from build123d import *

# Parameters (mm, degrees)
SKETCH1_R           = 125
SKETCH1_W           = 175
SKETCH1_H           = 95
BOSS_EXTRUDE1_DEPTH = 3
SKETCH2_R           = 3.25
SKETCH2_R_2         = 3
CUT_EXTRUDE1_DEPTH  = 4


with BuildPart() as part:
    # Sketch1 → Boss-Extrude1 (new body)
    with BuildSketch(Plane.XY):
        Circle(SKETCH1_R)
        Rectangle(SKETCH1_W, SKETCH1_H, mode=Mode.SUBTRACT)
    extrude(amount=BOSS_EXTRUDE1_DEPTH)

    # Sketch2 → Cut-Extrude1 (cut, through all)
    with BuildSketch(Plane.XY.offset(3)):
        with Locations((-52, -64.5)):
            Circle(SKETCH2_R)
        with Locations((-55, -93.5)):
            Circle(SKETCH2_R_2)
        with Locations((52, 64.5)):
            Circle(SKETCH2_R)
        with Locations((55, 93.5)):
            Circle(SKETCH2_R_2)
        with Locations((52, -64.5)):
            Circle(SKETCH2_R)
        with Locations((-52, 64.5)):
            Circle(SKETCH2_R)
        with Locations((49, -93.5)):
            Circle(SKETCH2_R)
        with Locations((-49, 93.5)):
            Circle(SKETCH2_R)
    extrude(amount=-CUT_EXTRUDE1_DEPTH, mode=Mode.SUBTRACT)


solid = part.part
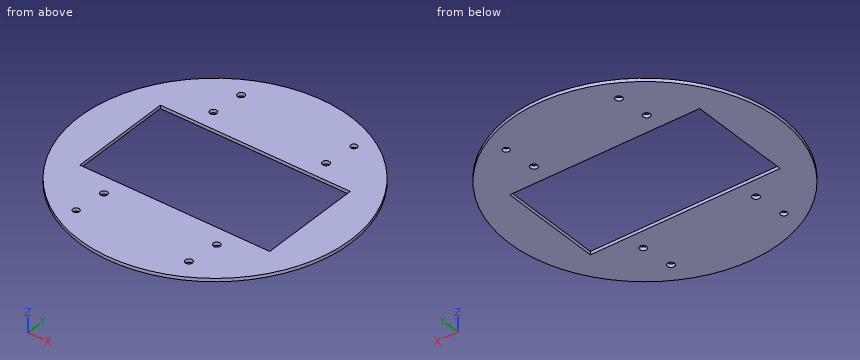
Part model, mm, in its own coordinate system. Give positions to 0.01 mm unless a question says otherwise; leave off trailing zeros. Loops run counter-clockwise (first coordinate to the right, second up) from the corner with the lowest first, then second, coordinate; pieces in that order, holes last.
(1) Band-saw the part on D-D (y = 93.5). Write the cut outline in (x, z), and give its area (3 significant figures).
Return value:
outline: (-82.96, 0) - (-52.25, 0) - (-52.25, 3) - (-82.96, 3) - close; (-45.75, 0) - (52, 0) - (52, 3) - (-45.75, 3) - close; (58, 0) - (82.96, 0) - (82.96, 3) - (58, 3) - close
area: 460 mm2
(2) Drill centre lines: line 1 along Y through (x, z) = (-1.5, 0.3); line 2 along Y through (x, z) = (-55, 2.1); line 3 along Y through (x, z) = (55, 1.95). Where is each one in solid material? Low to high.
Return value:
line 1: y = -124.99 to -47.5, 47.5 to 124.99
line 2: y = -112.25 to -96.5, -90.5 to -65.75, -63.25 to -47.5, 47.5 to 63.25, 65.75 to 112.25
line 3: y = -112.25 to -65.75, -63.25 to -47.5, 47.5 to 63.25, 65.75 to 90.5, 96.5 to 112.25
(3) Band-saw the part on B-B (z = 2). Count the separate pieces of the cut face and the enclosed holes in it, and give its area (3 significant figures).
Return value:
separate pieces: 1
enclosed holes: 9
area: 32,200 mm2
(4) Band-saw the part on A-A (y = 44). Write the cut outline in (x, z), and give its area (3 significant figures).
Return value:
outline: (-117, 0) - (-87.5, 0) - (-87.5, 3) - (-117, 3) - close; (87.5, 0) - (117, 0) - (117, 3) - (87.5, 3) - close
area: 177 mm2
(5) Pin check, flat tips, straight feed: pin 1 (4 mm diameter, centred on x = -52, y = 64.5, fed in from -Z) (3 decimals); pin 2 (3 mm diameter, centred on x = 77.5, y = 60, fed in from -Z); pin 3 (1.5 mm diameter, centred on y = -13, z = 1, fed in from +X); pin 4 (0.9 mm diameter, centred on x = -8, z = 1, fed in from -Y). Stop position of each tip, or through.
Return value:
pin 1: passes through
pin 2: stops at z = 0
pin 3: stops at x = 124.4
pin 4: stops at y = -124.77
(6) Band-saw the part on C-C (x = -33). Write the cut outline in (y, z).
Return value:
outline: (-120.57, 0) - (-47.5, 0) - (-47.5, 3) - (-120.57, 3) - close; (47.5, 0) - (120.57, 0) - (120.57, 3) - (47.5, 3) - close
